```python
from build123d import *

# Parameters (mm, degrees)
IZIM1_R                     = 35
Y_KSEKLIK_EKSTR_ZYON1_DEPTH = 600
IZIM2_R                     = 30
Y_KSEKLIK_EKSTR_ZYON2_DEPTH = 60


with BuildPart() as part:
    # Çizim1 → Yükseklik-Ekstrüzyon1 (new body)
    with BuildSketch(Plane.XY):
        Circle(IZIM1_R)
    extrude(amount=Y_KSEKLIK_EKSTR_ZYON1_DEPTH)

    # Çizim2 → Yükseklik-Ekstrüzyon2 (add, symmetric)
    with BuildSketch(Plane(origin=(0, 0, 0), x_dir=(1, 0, 0), z_dir=(0, 1, 0))):
        with BuildLine():
            Line((10, 0), (10, 11.270166538))
            ThreePointArc((10, 11.270166538), (0, 90), (-10, 11.270166538))
            Line((-10, 11.270166538), (-10, 0))
            Line((-10, 0), (10, 0))
        make_face()
        with Locations(Location((0, 50, 0), (0, 0, 270))):
            Circle(IZIM2_R, mode=Mode.SUBTRACT)
    extrude(amount=Y_KSEKLIK_EKSTR_ZYON2_DEPTH, both=True)


solid = part.part
```
Model file for the job. Use its own axes, mm. A direction names the side the tool comes from. Round coordinates to 2 decimals unless told otherwise and drop trailing zeros. Write each loop counter-clockwise with the first axis right and the second up, starting at its lowest first coordinate (ties: lowest second). Pieces come first, ordered by that corner, then holes. Notation, with made-up numbers: (71, 75) - (123, 75) arc R25 cw to (123, 103) - close; hole circle Ø3 at (28.25, 48.25). An arc over 180 degrees is marked (long way). Use CSV: the item, a comma, the result in double quotes. Start each with the question number.
Item 1: Band-saw the part on D-D (y = 47). Write the cut outline in (x, z).
Item 2: Band-saw the part on C-C (y = -6.5). Write the cut outline in (x, z).
Item 3: Drill centre lines: L1, parallel to Z at x = 1, y = -42; L2, parallel to X at y = 12, z = -50; L3, parallel to Z at x = -17, y = 29. Where is each one in solid material? Low to high. Write a range as [from, to].
Item 4: Two-plate mould, pull along Z, no slides. Class faces 4 (the face through (-10, 1, -6)), 5 (the face through (0, 0, 600)), 6 (the face through (-28, -21, 296)): released by +Z, released by -Z, zero draft, split by the parting line, or undercut.
Item 5: Pin check, flat tips, straight feed: P1, Ø6, axis at y = 22, z = 290, coming from the +X side; P2, Ø5.5, axis at y = 15, z = -5.5, coming from the -X side; P3, Ø5, axis at x = -14.5, z = 388, coming from the +Y side. Stop position of each tip, or through.
Item 6: Band-saw the part on B-B (x = 0). Write the cut outline in (y, z), and give its area (3 significant figures).
Item 7: Band-saw the part on A-A (z = -50). Write the cut outline in (x, y), and give its area (3 significant figures).
Item 8: Tool access for faces 1 (the face through (10, 1, -6)), 2 (the face through (1.32, -0.84, -79.97)), 3 (the face through (-20, 0, 0)): list every direction of +Z, -Z, +X, -X, +Y, -Y with a clear straight run to the whole face (end or side of a thin tool).
Checked values:
1,outline,"(-10, -11.27) arc R40 ccw (long way) to (10, -11.27) - (10, 0) - (-10, 0) - close; hole circle Ø60 at (0, -50)"
2,outline,"(-34.39, 0) - (-10, 0) - (-10, -11.27) arc R40 ccw (long way) to (10, -11.27) - (10, 0) - (34.39, 0) - (34.39, 600) - (-34.39, 600) - close; hole circle Ø60 at (0, -50)"
3,L1,"z = [-89.99, -79.98], [-20.02, 0]"
3,L2,"x = [-40, -30], [30, 40]"
3,L3,"z = [-86.21, -74.72], [-25.28, -13.79], [0, 600]"
4,face 4,"undercut"
4,face 5,"released by +Z"
4,face 6,"zero draft"
5,P1,"stops at x = 29.39"
5,P2,"stops at x = -10"
5,P3,"stops at y = 32.88"
6,outline,"(-60, -90) - (60, -90) - (60, -80) - (-60, -80) - close; (-60, -20) - (60, -20) - (60, 0) - (35, 0) - (35, 600) - (-35, 600) - (-35, 0) - (-60, 0) - close"
6,area,"45,600 mm²"
7,outline,"(-40, -60) - (-30, -60) - (-30, 60) - (-40, 60) - close; (30, -60) - (40, -60) - (40, 60) - (30, 60) - close"
7,area,"2,400 mm²"
8,face 1,"+X, +Y, -Y"
8,face 2,"+Y, -Y"
8,face 3,"-X, +Y, -Y"
